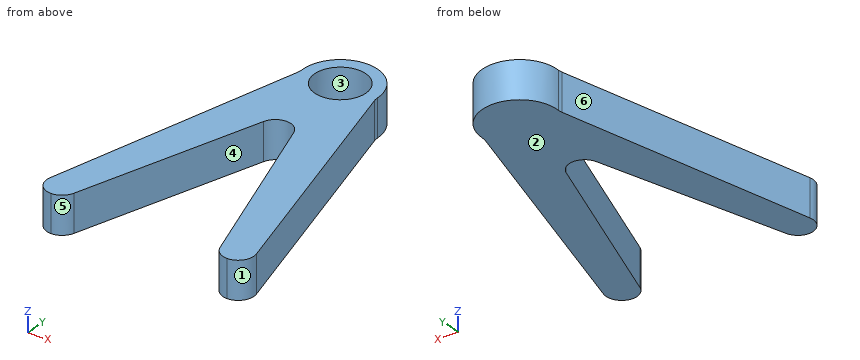
```python
from build123d import *

# Parameters (mm, degrees)
F0_R        = 8.2
F1_DEPTH    = 12
F2_DEPTH    = 2
F3_T1_DEPTH = 12
F3_T3_DEPTH = 30.2772195225
F3_T5_DEPTH = 44.2039362688


# Not quite as in the source:
# - a fillet or chamfer that OpenCascade refuses, or shapes differently, is made with other operations: its cross-section is extruded or revolved along the edge and cut away or added


with BuildPart() as f1:
    # F0 (on Top) → F1 (new body)
    with BuildSketch(Plane.XY):
        with BuildLine():
            Line((34.2691161265, 0), (11.9548385252, 87.1898676173))
            ThreePointArc((11.9548385252, 87.1898676173), (0, 100.2299809946), (-11.9548385252, 87.1898676173))
            Line((-11.9548385252, 87.1898676173), (-34.2691161265, 0))
            Line((-34.2691161265, 0), (-24.2691161265, 0))
            Line((-24.2691161265, 0), (0, 76.2299809946))
            Line((0, 76.2299809946), (24.2691161265, 0))
            Line((24.2691161265, 0), (34.2691161265, 0))
        make_face()
        with Locations((0, 88.2299809946)):
            Circle(F0_R, mode=Mode.SUBTRACT)
    extrude(amount=F1_DEPTH)

    # F0 (on Top) → F2 (join)
    with BuildSketch(Plane.XY):
        with Locations((0, 88.2299809946)):
            Circle(F0_R)
    extrude(amount=F2_DEPTH)

    # F3: fillet of radius 5 on 7 edges, made by hand

    # F3_s2 → F3_t1 (join)
    with BuildSketch(Plane.XY):
        with BuildLine():
            ThreePointArc((-4.7643738122, 61.2649479353), (0, 64.7481281774), (4.7643738122, 61.2649479353))
            Line((4.7643738122, 61.2649479353), (0, 76.2299809946))
            Line((0, 76.2299809946), (-4.7643738122, 61.2649479353))
        make_face()
        with BuildLine():
            ThreePointArc((11.9936747891, 87.8404106503), (12.0207340622, 87.1339702047), (12.1471577503, 86.4384075845))
            Line((12.1471577503, 86.4384075845), (11.9548385252, 87.1898676173))
            ThreePointArc((11.9548385252, 87.1898676173), (11.9786737183, 87.5148754431), (11.9936747891, 87.8404106503))
        make_face()
        with BuildLine():
            ThreePointArc((-12.1471577503, 86.4384075845), (-12.0207340622, 87.1339702047), (-11.9936747891, 87.8404106503))
            ThreePointArc((-11.9936747891, 87.8404106503), (-11.9786737183, 87.5148754431), (-11.9548385252, 87.1898676173))
            Line((-11.9548385252, 87.1898676173), (-12.1471577503, 86.4384075845))
        make_face()
    extrude(amount=F3_T1_DEPTH)

    # F3_s4 → F3_t3 (cut)
    with BuildSketch(Plane.XY.offset(-9.1386097613)):
        with BuildLine():
            ThreePointArc((-27.924560031, 0), (-24.9736363442, 0.96365891), (-23.1601862189, 3.4831802421))
            Line((-23.1601862189, 3.4831802421), (-24.2691161265, 0))
            Line((-24.2691161265, 0), (-27.924560031, 0))
        make_face()
        with BuildLine():
            ThreePointArc((23.1601862189, 3.4831802421), (24.9736363442, 0.96365891), (27.924560031, 0))
            Line((27.924560031, 0), (24.2691161265, 0))
            Line((24.2691161265, 0), (23.1601862189, 3.4831802421))
        make_face()
    extrude(amount=F3_T3_DEPTH, mode=Mode.SUBTRACT)

    # F3_s6 → F3_t5 (cut)
    with BuildSketch(Plane.XY.offset(-16.1019681344)):
        with BuildLine():
            ThreePointArc((-27.8283288728, 0), (-31.7779117903, 1.9339284455), (-32.6722104071, 6.239682089))
            Line((-32.6722104071, 6.239682089), (-34.2691161265, 0))
            Line((-34.2691161265, 0), (-27.8283288728, 0))
        make_face()
        with BuildLine():
            ThreePointArc((27.8283288728, 0), (31.7779117903, 1.9339284455), (32.6722104071, 6.239682089))
            Line((32.6722104071, 6.239682089), (34.2691161265, 0))
            Line((34.2691161265, 0), (27.8283288728, 0))
        make_face()
    extrude(amount=F3_T5_DEPTH, mode=Mode.SUBTRACT)


solid = f1.part
```
For this review, take the finished solid that the model builds, in its own axes (mm). Face numbers are marked on the shaded views. A direction names the side the tool comes from. Coordinates: 2 decimals unless noted, no trailing zeros. Loops run counter-clockwise (first coordinate to the right, second up) from the corner with the lowest first, then second, coordinate; pieces in that order, holes last.
1. Mouldability with a two-part tool opening along X and no side actions: class the marked faces 1, 2, 3 and 4 as +X half, -X half, draft (parallel to the pull), parting line (faces both ways), or undercut.
2. Add section D-D, the plane y = 77. Give the boundary of the cut face in (x, z).
3. For the marked faces 5 and 6, list the 3-axis set-ups (+Z, -Z, +X, -X, +Y, -Y) from which the entire face can be reached by the end or side of a thin tool; tool diameter is ignored.
4. Insertion check: P1, Ø1, axis at y = 16.5, z = 5.5, coming from the -X side; P2, Ø1.5, axis at y = 29, z = 9, coming from the -X side; P3, Ø3, axis at y = 67.5, z = 2.5, coming from the +X side. Each pin has a flat end and moves straight along its axis. Give the tip position at first contact, or say it passes through.
5. Add section B-B, the plane x = 0. Give the boundary of the cut face in (y, z).
6. Add section A-A, the plane y = 45.5. Give the boundary of the cut face in (x, z).
7. Add section C-C, the plane z = 5.75. Give the boundary of the cut face in (x, y).
8. For line 1 (Y direction, x = 0, z = 9); line 2 (X direction, y = 32, z = 1.5); line 3 (X direction, y = 90.5, z = 10.75), list the stretches that pass through material, from the lowest coordinate up.
Result:
1. face 1: +X half
1. face 2: draft
1. face 3: undercut
1. face 4: undercut
2. outline: (-14.56, 0) - (14.56, 0) - (14.56, 12) - (-14.56, 12) - close
3. face 5: +Z, -Z, -Y
3. face 6: +Z, -Z, -X, +Y
4. P1: stops at x = -30.17
4. P2: stops at x = -27.04
4. P3: stops at x = 17.38
5. outline: (64.75, 0) - (100.23, 0) - (100.23, 12) - (96.43, 12) - (96.43, 2) - (80.03, 2) - (80.03, 12) - (64.75, 12) - close
6. outline: (-22.62, 0) - (-9.78, 0) - (-9.78, 12) - (-22.62, 12) - close; (9.78, 0) - (22.62, 0) - (22.62, 12) - (9.78, 12) - close
7. outline: (-32.67, 6.24) arc R5 ccw to (-27.88, 0) arc R5 ccw to (-23.16, 3.48) - (-4.76, 61.26) arc R5 cw to (4.76, 61.26) - (23.16, 3.48) arc R5 ccw to (27.88, 0) arc R5 ccw to (32.67, 6.24) - (12.15, 86.44) arc R5 cw to (11.99, 87.84) arc R12 ccw (long way) to (-11.99, 87.84) arc R5 cw to (-12.15, 86.44) - close; hole circle Ø16.4 at (0, 88.23)
8. line 1: y = 64.75 to 80.03, 96.43 to 100.23
8. line 2: x = -26.08 to -14.08, 14.08 to 26.08
8. line 3: x = -11.78 to -7.88, 7.88 to 11.78
